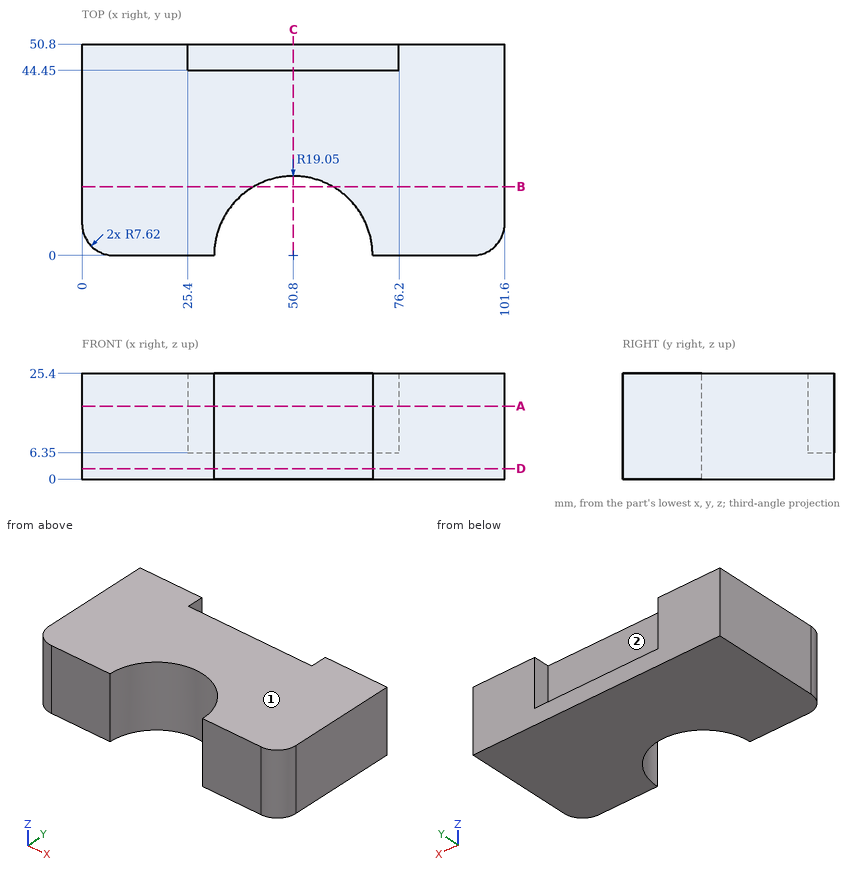
Design review of the part shown in the three views and the two pictorial views. Dimensions are in mm from the part's minimum x, y and z. A direction names the side the tool comes from. Coordinates: 2 decimals unless noted, no trailing zeros. Order: outer loops, then holes, each group sorted by start corner. A loop starts at its lowest first (then second) coordinate and runs counter-clockwise, first axis right, second up. Notation, with made-up numbers: (-31.75, 20) - (-5.75, 20) arc R11 ccw to (-5.75, 32) - close; hole circle Ø4 at (59.5, -3). An arc over 180 degrees is marked (long way). One line per question, with ' | ' between items.
Q1. Consider section C-C, the plane x = 50.8. Give the boundary of the cut face in (y, z), then the cut area to 3 significant figures.
Answer key:
outline: (19.05, 0) - (50.8, 0) - (50.8, 6.35) - (44.45, 6.35) - (44.45, 25.4) - (19.05, 25.4) - close | area: 685 mm2
Q2. For the marked faces 1 and 2, list the 3-axis set-ups (+Z, -Z, +X, -X, +Y, -Y) from which the entire face can be reached by the end or side of a thin tool; tool diameter is ignored.
Answer key:
face 1: +Z, +X, -X, +Y, -Y | face 2: +Z, +Y
Q3. To check wall thickness, follow line 1 along X through (y, z) = (3.5, 19.5); line 2 along X through (y, z) = (44.5, 23.25); line 3 along Z through (x, y) = (46, 48.5). State the ranges of each line that lie inside material, in increasing order.
Answer key:
line 1: x = 1.21 to 32.07, 69.53 to 100.39 | line 2: x = 0 to 25.4, 76.2 to 101.6 | line 3: z = 0 to 6.35
Q4. Clearance check with flat-ended pins moving along their axes: pin 1 Ø1.5 at (x, z) = (54, 8.5) entering from -Y; pin 2 Ø1 at (x, z) = (47.5, 6.5) entering from -Y; pin 3 Ø8 at (x, z) = (49, 21.5) entering from +Y. State where each tip first meets the part, or that it passes through.
Answer key:
pin 1: stops at y = 18.64 | pin 2: stops at y = 18.67 | pin 3: stops at y = 44.45
Q5. Consider section A-A, the plane z = 17.5. Give the boundary of the cut face in (x, y), then the cut area to 3 significant figures.
Answer key:
outline: (0, 7.62) arc R7.62 ccw to (7.62, 0) - (31.75, 0) arc R19.05 cw to (69.85, 0) - (93.98, 0) arc R7.62 ccw to (101.6, 7.62) - (101.6, 50.8) - (76.2, 50.8) - (76.2, 44.45) - (25.4, 44.45) - (25.4, 50.8) - (0, 50.8) - close | area: 4,240 mm2
Q6. Consider section B-B, the plane y = 16.5. Give the boundary of the cut face in (x, z).
Answer key:
outline: (0, 0) - (41.28, 0) - (41.28, 25.4) - (0, 25.4) - close; (60.32, 0) - (101.6, 0) - (101.6, 25.4) - (60.32, 25.4) - close
Q7. Consider section D-D, the plane z = 2.5. Give the boundary of the cut face in (x, y).
Answer key:
outline: (0, 7.62) arc R7.62 ccw to (7.62, 0) - (31.75, 0) arc R19.05 cw to (69.85, 0) - (93.98, 0) arc R7.62 ccw to (101.6, 7.62) - (101.6, 50.8) - (0, 50.8) - close
